Autodesk Inventor part; units mm, degrees
ref_plane "YZ Plane" through (0, 0, 0) normal (1, 0, 0) x (0, 1, 0)
ref_plane "XZ Plane" through (0, 0, 0) normal (0, 1, 0) x (-1, 0, 0)
ref_plane "XY Plane" through (0, 0, 0) normal (0, 0, 1) x (1, 0, 0)
sketch "Sketch1" plane through (0, 0, 0) normal (0, 0, 1) x (1, 0, 0)
  line L0 (0, 0) -> (63.5, 0)
  line L1 (63.5, 0) -> (63.5, 31.75)
  line L2 (63.5, 31.75) -> (0, 31.75)
  line L3 (0, 31.75) -> (0, 0)
  dimension "d0" = 63.5
  dimension "d1" = 31.75
extrude "Extrusion1" add sketch "Sketch1" along normal blind 12.7
sketch "Sketch2" plane through (0, 0, 12.7) normal (0, 0, 1) x (1, 0, 0)
  line L0 (63.5, 0) -> (63.5, 31.75)
  line L1 (63.5, 12.7901) -> (80.6196, 12.7901) construction
  line L2 (0, 0) -> (63.5, 0)
  line L3 (46.3804, 0) -> (46.3804, 14.605)
  line L4 (46.3804, 0) -> (60.9854, 0) construction
  circle A0 centre (46.3804, 14.605) radius 3.4925
  circle A1 centre (46.3804, 14.605) radius 8.001
  circle A2 centre (46.3804, 6.604) radius 1.5875
  circle A3 centre (53.3095, 10.6045) radius 1.5875
  circle A4 centre (46.3804, 14.605) radius 8.001
  circle A5 centre (53.3095, 18.6055) radius 1.5875
  circle A6 centre (46.3804, 14.605) radius 8.001
  circle A7 centre (46.3804, 22.606) radius 1.5875
  circle A8 centre (46.3804, 14.605) radius 8.001
  circle A9 centre (39.4513, 18.6055) radius 1.5875
  circle A10 centre (46.3804, 14.605) radius 8.001
  circle A11 centre (39.4513, 10.6045) radius 1.5875
  circle A12 centre (46.3804, 14.605) radius 8.001
  dimension "d9" = 16.002
  dimension "d6" = 14.605
  dimension "d7" = 90
  dimension "d8" = 6.985
  dimension "d10" = 3.175
  dimension "d13" = 360
  dimension "d17" = 17.1196
extrude "Extrusion2" cut sketch "Sketch2" against normal blind 19.05 contours A2 A1 L3 | L3 A1 A2 | A1 A2 L3 | L3 A2 A1 | A11 A1 | A1 A11 | A3 A1 | A1 A3 | A9 A1 | A1 A9 | A5 A1 | A1 A5 | A7 A1 | A1 A7 | A0
thicken "Thicken1" operation add thickness 25.4 both sides no extend neighbours yes toward (-1, 0, 0) faces at (0, 21.1667, 4.2333)
sketch "Sketch4" plane through (63.5, 0, 0) normal (0, -1, 0) x (1, 0, 0)
  line L0 (-88.9, 0) -> (-88.9, 12.7)
  line L1 (0, 0) -> (0, 12.7)
  point P0 (-63.5, 0)
  point P1 (-82.55, 6.35)
  point P2 (-44.45, 6.35)
  point P3 (-6.35, 6.35)
  dimension "d42" = 6.35
  dimension "d43" = 88.9
  dimension "d44" = 44.45
  dimension "d45" = 6.35
hole "Hole1" at (-19.05, 0, 6.35) at (19.05, 0, 6.35) at (57.15, 0, 6.35) direction (0, 1, 0) diameter 3.302 depth 7.62 tip angle 118
properties part number "MotorHolderB"
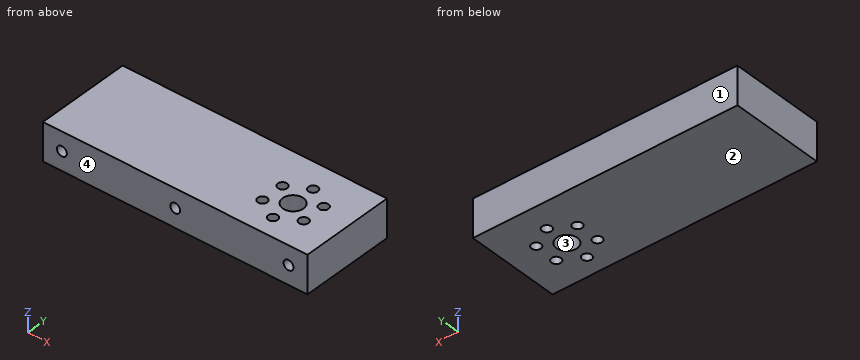
For this review, take the finished solid that the model builds, in its own axes (mm). Face numbers are marked on the shaded views. Round coordinates to 2 decimals unless told otherwise and drop trailing zeros. Write each loop counter-clockwise with the first axis right and the second up, starting at its lowest first coordinate (ties: lowest second). Pieces come first, ordered by that corner, then holes. Notation, with made-up numbers: (30.5, 83) -> (59.5, 83) arc R25 cw to (59.5, 106) -> close; hole circle Ø9 at (-23.75, 82.5). An arc over 180 degrees is marked (long way). Put each result on its own line as item: value.
Q1. The part is to be moulded in two halves that separate along Y. For the marked faces 1, 2, 3 and 4, say which applies: released by +Y, released by -Y, zero draft, split by the parting line, or undercut.
Determined:
face 1: released by +Y
face 2: zero draft
face 3: undercut
face 4: released by -Y
Q2. Consider section B-B on z = 2.75. Give the number of separate pieces and of enclosed holes in the cut face, and give its area (3 significant figures).
Determined:
separate pieces: 1
enclosed holes: 7
area: 2,740 mm^2
Q3. Consider section A-A on y = 4. State the section outline as (x, z) points.
Determined:
outline: (-25.4, 0) -> (63.5, 0) -> (63.5, 12.7) -> (-25.4, 12.7) -> close; hole circle Ø3.3 at (-19.05, 6.35); hole circle Ø3.3 at (19.05, 6.35); hole circle Ø3.3 at (57.15, 6.35)
Q4. To check wall thickness, follow L1, parallel to X at y = 2.75, z = 6.35; L2, parallel to Z at x = 57.15, y = 5.25; L3, parallel to X at y = 6, z = 6.35. State the ranges of each line that lie inside material, in increasing order. Write a range as [from, to].
Determined:
L1: x = [-25.4, -20.7], [-17.4, 17.4], [20.7, 55.5], [58.8, 63.5]
L2: z = [0, 4.7], [8, 12.7]
L3: x = [-25.4, -20.7], [-17.4, 17.4], [20.7, 44.91], [47.85, 55.5], [58.8, 63.5]
